```python
from build123d import *

# Parameters (mm, degrees)
SKETCH1_R           = 5.35
SKETCH4_R           = 7.25
BOSS_EXTRUDE1_DEPTH = 9.8
BOSS_EXTRUDE1_TAPER = 2
SHELL1_T            = -2
SKETCH7_R           = 0.5
CIRPATTERN1_COUNT   = 8
SKETCH8_R           = 5.8
CUT_EXTRUDE1_DEPTH  = 2.8
SKETCH9_W           = 9.16
SKETCH9_H           = 2
CUT_EXTRUDE2_DEPTH  = 50.87283838
BOSS_EXTRUDE2_DEPTH = 1.5
SKETCH11_R          = 1.9
BOSS_EXTRUDE3_DEPTH = 1.5


with BuildPart() as part:
    # Base-Sweep: sweep along a path in Sketch2
    with BuildLine(Plane.XY) as base_sweep_path:
        Line((0, 6.4), (0, 8.9))
        ThreePointArc((0, 8.9), (-2.987510832, 16.112489168), (-10.2, 19.1))
        Line((-10.2, 19.1), (-25.4, 19.1))
    # Sketch1 → Base-Sweep (sweep)
    with BuildSketch(Plane(origin=(0, 6.4, 0), x_dir=(-1, 0, 0), z_dir=(0, 1, 0))):
        Circle(SKETCH1_R)
    sweep(path=base_sweep_path.line)

    # Sketch3 → Boss-Revolve1 (revolve)
    with BuildSketch(Plane.XY, mode=Mode.PRIVATE) as boss_revolve1_sk:
        with BuildLine():
            Line((-27.412489016, 28), (-30.5, 28))
            Line((-30.5, 28), (-30.5, 19.1))
            Line((-30.5, 19.1), (-18.512489016, 19.1))
            ThreePointArc((-18.512489016, 19.1), (-21.119238663, 25.393250353), (-27.412489016, 28))
        make_face()
    revolve(boss_revolve1_sk.sketch.rotate(Axis((-36.172167942, 19.1, 0), (-1, 0, 0)), 270), axis=Axis((-36.172167942, 19.1, 0), (-1, 0, 0)))

    # Sketch4 → Boss-Extrude1 (add)
    with BuildSketch(Plane.ZY.offset(30.5)):
        with Locations((0, 19.1)):
            Circle(SKETCH4_R)
    extrude(amount=BOSS_EXTRUDE1_DEPTH, taper=BOSS_EXTRUDE1_TAPER)

    # Shell1
    shell1_openings = [part.faces().sort_by_distance(p)[0] for p in [
        (-40.3, 19.1, 0),
        (0, 6.4, 0),
    ]]
    offset(amount=SHELL1_T, openings=shell1_openings, kind=Kind.INTERSECTION)

    # Boss-Sweep1: sweep along a path in Sketch6
    with BuildLine(Plane(origin=(0, 2.79713024, 6.75286976), x_dir=(1, 0, 0), z_dir=(0, 0.38268343236509056, 0.9238795325112865))) as boss_sweep1_path:
        Line((-36.9, 24.672606146), (-30.5, 24.896099071))
    # Sketch7 → Boss-Sweep1 (sweep)
    with BuildSketch(Plane.ZY.offset(30.5)):
        with Locations((-2.621381512, 25.428574798)):
            Circle(SKETCH7_R)
    boss_sweep1 = sweep(path=boss_sweep1_path.line)

    # CirPattern1: Boss-Sweep1 ×8 about axis
    cirpattern1_axis = Axis((-36.172167942, 19.1, 0), (-1, 0, 0))
    for i in range(1, CIRPATTERN1_COUNT):
        add(boss_sweep1.rotate(cirpattern1_axis, i * 360 / CIRPATTERN1_COUNT))

    # Sketch8 → Cut-Extrude1 (cut)
    with BuildSketch(Plane.ZY.offset(40.3)):
        with Locations(Location((0, 19.1, 0), (0, 0, 270))):
            Circle(SKETCH8_R)
    extrude(amount=-CUT_EXTRUDE1_DEPTH, mode=Mode.SUBTRACT)

    # Sketch9 → Cut-Extrude2 (cut, through all)
    with BuildSketch(Plane(origin=(0, 0, 0), x_dir=(1, 0, 0), z_dir=(0, 1, 0))):
        with Locations((-35.72, 0)):
            Rectangle(SKETCH9_W, SKETCH9_H)
    extrude(amount=CUT_EXTRUDE2_DEPTH, mode=Mode.SUBTRACT)

    # Sketch10 → Boss-Extrude2 (add)
    with BuildSketch(Plane(origin=(0, 12.319, -3.6), x_dir=(1, 0, 0), z_dir=(0, 0, -1))):
        with BuildLine():
            Line((-4.95, 5.919), (4.95, 5.919))
            Line((4.95, 5.919), (4.95, 11.869))
            ThreePointArc((4.95, 11.869), (0, 16.819), (-4.95, 11.869))
            Line((-4.95, 11.869), (-4.95, 5.919))
        make_face()
    boss_extrude2 = extrude(amount=-BOSS_EXTRUDE2_DEPTH)

    # Sketch11 → Boss-Extrude3 (add)
    with BuildSketch(Plane(origin=(0, 0, -3.6), x_dir=(-1, 0, 0), z_dir=(0, 0, -1))):
        with Locations(Location((0, 0, 0), (0, 0, 180))):
            Circle(SKETCH11_R)
    boss_extrude3 = extrude(amount=BOSS_EXTRUDE3_DEPTH)

    # Mirror1: Boss-Extrude2, Boss-Extrude3 across plane
    add(boss_extrude2.mirror(Plane.XY))
    add(boss_extrude3.mirror(Plane.XY))


solid = part.part
```
For this review, take the finished solid that the model builds, in its own axes (mm). A direction names the side the tool comes from. Round coordinates to 2 decimals unless told otherwise and drop trailing zeros. Write each loop counter-clockwise with the first axis right and the second up, starting at its lowest first coordinate (ties: lowest second). Pieces come first, ordered by that corner, then holes. Notation, with made-up numbers: (3.5, 70) - (34.5, 70) arc R14 ccw to (34.5, 92) - close; hole circle Ø10 at (78, -30). An arc over 180 degrees is marked (long way). Answer as a JSON object with one key per item and string values.
1. Tool access review of faces 4 (the face through (-38.9, 19, 5.8)), 5 (the face through (1.812, -0.571, 4.34)), 6 (the face through (0, 1, -2.1)), 7 (the face through (-4.95, 3, 3)): name each direction out of +Z, -Z, +X, -X, +Y, -Y from which nothing blocks a thin tool from reaching the whole face with its end or side.
Response values:
{"face 4": "-X", "face 5": "+Z", "face 6": "+X, -X, -Y", "face 7": "+Z, -Z, -X, -Y"}
2. To check wall thickness, follow line 1 along Y through (x, z) = (-18, 0); line 2 along Z through (x, y) = (-4.5, 2); line 3 along Y through (x, z) = (-28, 0). State the ranges of each line that lie inside material, in increasing order.
Response values:
{"line 1": "y = 13.75 to 15.75, 22.45 to 24.45", "line 2": "z = -3.6 to -2.1, 2.1 to 3.6", "line 3": "y = 10.2 to 12.2, 26 to 28"}
3. We need section C-C on x = -25.5. Give the boundary of the cut face in (y, z), then the cut area to 3 significant figures.
Response values:
{"outline": "circle Ø17.38 at (19.1, 0); hole circle Ø13.26 at (19.1, 0)", "area": "99.3 mm2"}
4. Draft analysis for pull direction Y (two halves, no side actions). For faces 1 (the face through (-0.1, 2.1, 3.6)), 2 (the face through (0, 1, 2.1)), 3 (the face through (4.7, 6.4, 3.2)), state which applies: +Y half, -Y half, draft (parallel to the pull), parting line (faces both ways), or undercut.
Response values:
{"face 1": "undercut", "face 2": "draft", "face 3": "+Y half"}
5. For pin 1 Ø2 at (y, z) = (7.5, -5) entering from -X; pin 2 Ø4 at (x, y) = (-8.5, 12.5) entering from -Z; pin 3 Ø0.8 at (y, z) = (3, 2.5) entering from +X, all flat-tipped, find the tip position at first contact; note any pin that passes through.
Response values:
{"pin 1": "stops at x = -3.55", "pin 2": "stops at z = -3.29", "pin 3": "stops at x = 4.95"}
6. We need section A-A on y = -1. Give the boundary of the cut face in (x, z).
Response values:
{"outline": "(-4.73, -3.6) - (-1.62, -3.6) - (-1.62, -5.1) - (1.62, -5.1) - (1.62, -3.6) - (4.73, -3.6) - (4.73, -2.1) - (-4.73, -2.1) - close; (-4.73, 2.1) - (4.73, 2.1) - (4.73, 3.6) - (1.62, 3.6) - (1.62, 5.1) - (-1.62, 5.1) - (-1.62, 3.6) - (-4.73, 3.6) - close"}
